Input: part model. Units: mm. Frame: model coordinates. A direction names the side the tool comes from. Give positions to 0.01 mm unless a question says otherwise; leave off trailing zeros. Order: outer loops, then holes, each group sorted by start corner. A loop starts at its lowest first (then second) coordinate and runs counter-clockwise, first axis right, second up. Notation, with made-up numbers: (25.25, -6.75) -> (69.25, -6.75) arc R14 cw to (69.25, 8.25) -> close; hole circle Ø6 at (33.25, 83.25). An arc over 180 degrees is marked (long way). Use a Markdown table: item, result. Add a question column.
Autodesk Inventor part; units mm, degrees
ref_plane "YZ Plane" through (0, 0, 0) normal (1, 0, 0) x (0, 1, 0)
ref_plane "XZ Plane" through (0, 0, 0) normal (0, 1, 0) x (-1, 0, 0)
ref_plane "XY Plane" through (0, 0, 0) normal (0, 0, 1) x (1, 0, 0)
sketch "スケッチ1" plane through (0, 0, 0) normal (0, 0, 1) x (1, 0, 0)
  circle A0 centre (0, 0) radius 4.25
  dimension "d0" = 8.5
extrude "押し出し1" add sketch "スケッチ1" against normal blind 23
sketch "スケッチ2" plane through (0, 0, 0) normal (0, 0, 1) x (1, 0, 0)
  circle A0 centre (0, 0) radius 0.5
  dimension "d3" = 1
extrude "押し出し2" add sketch "スケッチ2" along normal blind 4.8
sketch "スケッチ3" plane through (0, 0, 0) normal (0, 0, 1) x (1, 0, 0)
  circle A0 centre (0, 0) radius 0.5
  circle A1 centre (0, 0) radius 1
  dimension "d6" = 2
extrude "押し出し3" add sketch "スケッチ3" along normal blind 0.5
properties part number "8523Motor"
Q1. Section query D-D (x = 2.25). Return loops of the section in (y, z).
Q2. First-contact query: pin 1 (2.5 mm diameter, centred on x = -1, y = 1.5, fed in from +Z); pin 2 (1.5 mm diameter, centred on y = 1, z = -10, fed in from -X); pin 3 (3 mm diameter, centred on x = -2.5, y = -3, fed in from +Z). Flat tips, straight axial feed; report the tip coordinate or a pass-through.
Q3. Section query A-A (y = 0). Return loops of the section in (x, z).
Q4. Ray query, line 1 (Z direction, x = 1, y = 2); line 2 (X direction, y = -2, z = -2.25); line 3 (X direction, y = 2.25, z = -18). Return the intervals inside material, ascending.
Q5. Section query C-C (z = -20.5). Return loops of the section in (x, y), plus the area to 3 significant figures.
Q6. Access query for faces 1 (the cylindrical face through (2.285, 3.584, -11.339)), 2 (the cylindrical face through (-0.108, 0.488, 2.62)). Directions: +Z, -Z, +X, -X, +Y, -Y. A direction counts if a zero-diameter tool reaches every point of the face in a straight line with its end or side. Return the directions, or none.
Solution:
| question | item | result |
|---|---|---|
| 1 | outline | (-3.61, -23) -> (3.61, -23) -> (3.61, 0) -> (-3.61, 0) -> close |
| 2 | pin 1 | stops at z = 0.5 |
| 2 | pin 2 | stops at x = -4.24 |
| 2 | pin 3 | stops at z = 0 |
| 3 | outline | (-4.25, -23) -> (4.25, -23) -> (4.25, 0) -> (1, 0) -> (1, 0.5) -> (0.5, 0.5) -> (0.5, 4.8) -> (-0.5, 4.8) -> (-0.5, 0.5) -> (-1, 0.5) -> (-1, 0) -> (-4.25, 0) -> close |
| 4 | line 1 | z = -23 to 0 |
| 4 | line 2 | x = -3.75 to 3.75 |
| 4 | line 3 | x = -3.61 to 3.61 |
| 5 | outline | circle Ø8.5 at (0, 0) |
| 5 | area | 56.7 mm² |
| 6 | face 1 | +Z, -Z |
| 6 | face 2 | +Z |
